Source: CAD feature listing. Evaluate the final solid. Frame: model axes, mm. A direction names the side the tool comes from. Give positions to 0.01 mm unless a question says otherwise; leave off trailing zeros. Loops run counter-clockwise (first coordinate to the right, second up) from the corner with the lowest first, then second, coordinate; pieces in that order, holes last. Notation, with made-up numbers: (33, 87.5) -> (55, 87.5) arc R32 cw to (55, 125.5) -> close; hole circle Ø3 at (48, 0.5). An arc over 180 degrees is marked (long way). Return JSON: item names as keys, results as strings. Group by question number.
(1) Ray query, line 1 (X direction, y = -1.25, z = 4.75); line 2 (X direction, y = 1.75, z = 4.75); line 3 (X direction, y = -5, z = 2.75). Return the intervals inside material, ascending. Write a range as from..to.
(2) Cut plane A-A on z = 2.5. Return loops of the section in (x, y) (3 decimals).
(3) Draft query along X for faces 6 (the face through (-105.729, 4, 7)), 7 (the face through (-22, 5.919, 5)), 8 (the face through (46.66, -0.04, 2.54)). Return one class per face: released by +X, released by -X, zero draft, split by the parting line, or undercut.
(4) Access query for faces 1 (the face through (-110.659, 3.073, 4.93)), 2 (the face through (34.271, -2, 8)), 3 (the face through (-98.534, -5.383, 5.07)), 4 (the face through (-115.729, -2, 4)), 5 (the face through (-110.659, -6.154, 5.07)). Directions: +Z, -Z, +X, -X, +Y, -Y. A direction counts if a zero-diameter tool reaches every point of the face in a straight line with its end or side. Return the directions, or none.
(5) Pin query (flat end, axial travel): pin 1 (2.5 mm diameter, centred on y = 0, z = 7, fed in from +X); pin 2 (2 mm diameter, centred on x = -94.5, y = -3.5, fed in from +Z); pin 3 (7.5 mm diameter, centred on x = 47.5, y = -1, fed in from +Z). Return the tip coordinate at first contact, or that it passes through.
```python
from build123d import *

# Parameters (mm, degrees)
SKETCH_W        = 170
SKETCH_H        = 15
PAD_DEPTH       = 10
SKETCH001_W     = 35
SKETCH001_H     = 25
POCKET_DEPTH    = 5
PAD002_DEPTH    = 10
POCKET001_DEPTH = 10
SKETCH002_R     = 5.125
POCKET002_DEPTH = 5


with BuildPart() as part:
    # Sketch → Pad (new body)
    with BuildSketch(Plane.XY):
        with Locations((-20.728933, -1.58076)):
            Rectangle(SKETCH_W, SKETCH_H)
    extrude(amount=PAD_DEPTH)

    # Sketch001 (on Face6 of Pad) → Pocket (cut)
    with BuildSketch(Plane.XY.offset(10)):
        with Locations((51.771067, -1.58076)):
            Rectangle(SKETCH001_W, SKETCH001_H)
    extrude(amount=-POCKET_DEPTH, mode=Mode.SUBTRACT)

    # Sketch003 → Pad002 (join)
    with BuildSketch(Plane(origin=(-105.728933, 0, 0), x_dir=(0, -1, 0), z_dir=(-1, 0, 0))):
        Polygon((-5.91924, 0), (-0.145737, 10), (3.307257, 10), (9.08076, 0), align=None)
    extrude(amount=PAD002_DEPTH)

    # Sketch004 (on Face3 of Pad002) → Pocket001 (cut)
    with BuildSketch(Plane.XY.offset(10)):
        Polygon((-93.103933, -14.787648), (-100.728933, -1.58076), (-85.478933, -1.58076), align=None)
    extrude(amount=-POCKET001_DEPTH, mode=Mode.SUBTRACT)

    # Sketch002 (on Face7 of Pocket) → Pocket002 (cut)
    with BuildSketch(Plane.XY.offset(5)):
        with Locations((56.771067, -1.58076)):
            Circle(SKETCH002_R)
        with Locations((41.771067, -1.58076)):
            Circle(SKETCH002_R)
    extrude(amount=-POCKET002_DEPTH, mode=Mode.SUBTRACT)


solid = part.part
```
Answers:
{
 "1": {"line 1": "-115.73..36.66, 46.89..51.66, 61.89..64.27", "line 2": "-115.73..37.88, 45.67..52.88, 60.67..64.27", "line 3": "-115.73..-98.75, -87.45..37.95, 45.59..52.95, 60.59..64.27"},
 "2": {"outline": "(-115.729, -7.637) -> (-105.729, -7.637) -> (-105.729, -9.081) -> (-96.399, -9.081) -> (-100.729, -1.581) -> (-85.479, -1.581) -> (-89.809, -9.081) -> (64.271, -9.081) -> (64.271, 5.919) -> (-105.729, 5.919) -> (-105.729, 4.476) -> (-115.729, 4.476) -> close; hole circle Ø10.25 at (41.771, -1.581); hole circle Ø10.25 at (56.771, -1.581)"},
 "3": {"face 6": "released by -X", "face 7": "zero draft", "face 8": "undercut"},
 "4": {"face 1": "+Z, -X, +Y", "face 2": "+Z, +X, +Y, -Y", "face 3": "+Z, -Z", "face 4": "+Z, -Z, -X, +Y, -Y", "face 5": "+Z, -X, -Y"},
 "5": {"pin 1": "x = 34.27", "pin 2": "through", "pin 3": "z = 5"}
}
